For this review, take the finished solid that the model builds, in its own axes (mm). Face numbers are marked on the shaded views. Coordinates: 2 decimals unless noted, no trailing zeros. Loops run counter-clockwise (first coordinate to the right, second up) from the corner with the lowest first, then second, coordinate; pieces in that order, holes last. Notation, with made-up numbers: (32.25, 31.25) - (55.25, 31.25) arc R32 ccw to (55.25, 70.25) - close; hole circle Ø9 at (80.25, -37.75). An arc over 180 degrees is marked (long way). Answer as a JSON object with one key per item and string values. Group by question number.
Item 1: We need section B-B (z = -1.7). Give the boundary of the cut face in (x, y), then the cut area to 3 significant figures.
Item 2: Mouldability with a two-part tool opening along X and no side actions: class the marked faces 1, 2, 3 and 4 as released by +X, released by -X, zero draft, split by the parting line, or undercut.
Item 3: To check wall thickness, follow line 1 (Y direction, x = 0, z = -3); line 2 (Y direction, x = -5, z = -4.65); line 3 (X direction, y = -1.75, z = -4.35). State the ranges of each line that lie inside material, in increasing order.
Item 4: We need section A-A (x = 0). Give the boundary of the cut face in (y, z).
Item 5: We need section C-C (z = -3.3). Give the boundary of the cut face in (x, y), then the cut area to 3 significant figures.
Item 6: Clearance check with flat-ended pins moving along their axes: pin 1 (1.5 mm diameter, centred on y = 6, z = -5, fed in from +X); pin 2 (1.8 mm diameter, centred on x = 5, y = 0, fed in from -Z); pin 3 (1.5 mm diameter, centred on y = 6.5, z = -3.5, fed in from +X). State where each tip first meets the part, or that it passes through.
from build123d import *

# Parameters (mm, degrees)
F0_R     = 8
F2_DEPTH = 6
F3_D     = 6.8
F3_DEPTH = 13.8976
F3_TIP   = 2.0429261047
F4_SIZE  = 1.5
F6_D     = 2
F6_DEPTH = 3
F6_TIP   = 0.600860619


with BuildPart() as f2:
    # F0 (on Top) → F2 (new body)
    with BuildSketch(Plane.XY):
        Circle(F0_R)
    extrude(amount=-F2_DEPTH)

    # F3
    with Locations(Plane.XY):
        with Locations((0, 0)):
            Hole(F3_D / 2, depth=F3_DEPTH)
            with Locations((0, 0, -(F3_DEPTH + F3_TIP / 2))):  # 118° drill point
                Cone(0, F3_D / 2, F3_TIP, mode=Mode.SUBTRACT)

    # F4
    f4_edges = [f2.edges().sort_by_distance(p)[0] for p in [
        (-8, 0, -6),
    ]]
    chamfer(f4_edges, length=F4_SIZE)

    # F6
    with Locations(Plane(origin=(0, 0, -6), x_dir=(1, 0, 0), z_dir=(0, 0, -1))):
        with Locations((-5, 0), (5, 0)):
            Hole(F6_D / 2, depth=F6_DEPTH)
            with Locations((0, 0, -(F6_DEPTH + F6_TIP / 2))):  # 118° drill point
                Cone(0, F6_D / 2, F6_TIP, mode=Mode.SUBTRACT)


solid = f2.part
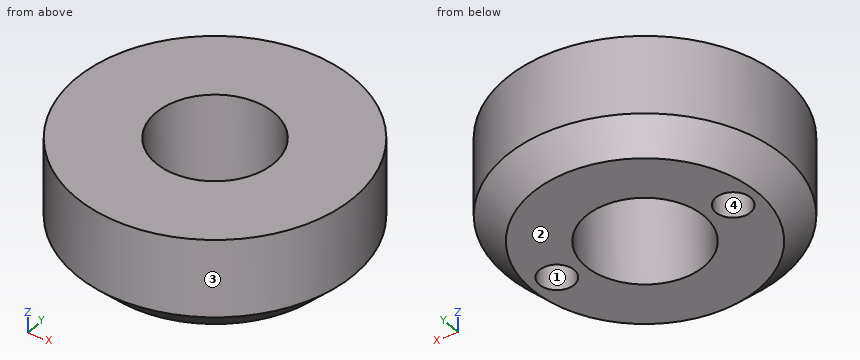
Check sheet entries:
{
 "1": {"outline": "circle Ø16 at (0, 0); hole circle Ø6.8 at (0, 0)", "area": "165 mm2"},
 "2": {"face 1": "undercut", "face 2": "zero draft", "face 3": "split by the parting line", "face 4": "undercut"},
 "3": {"line 1": "y = -8 to -3.4, 3.4 to 8", "line 2": "y = -6.05 to -1, 1 to 6.05", "line 3": "x = -7.81 to -2.92, 2.92 to 7.81"},
 "4": {"outline": "(-8, -4.5) - (-6.5, -6) - (-3.4, -6) - (-3.4, 0) - (-8, 0) - close; (3.4, -6) - (6.5, -6) - (8, -4.5) - (8, 0) - (3.4, 0) - close"},
 "5": {"outline": "circle Ø16 at (0, 0); hole circle Ø2 at (-5, 0); hole circle Ø6.8 at (0, 0); hole circle Ø2 at (5, 0)", "area": "158 mm2"},
 "6": {"pin 1": "stops at x = 5.86", "pin 2": "stops at z = -2.94", "pin 3": "stops at x = 5.56"}
}
